from build123d import *

# Parameters (mm, degrees)
BOSS_EXTRU_1_DEPTH                                 = 14
BOSS_EXTRU_1_DEPTH_BACK                            = 7
ESQUISSE1_R                                        = 115
ESQUISSE1_R_2                                      = 10
ESQUISSE1_R_3                                      = 15.264337522
CHAMBRAGE_POUR_VIS_T_TE_HEXAGONALE_M12_D           = 13.5
CHAMBRAGE_POUR_VIS_T_TE_HEXAGONALE_M12_DEPTH       = 20
CHAMBRAGE_POUR_VIS_T_TE_HEXAGONALE_M12_CBORE_D     = 20
CHAMBRAGE_POUR_VIS_T_TE_HEXAGONALE_M12_CBORE_DEPTH = 12.6
CHAMBRAGE_POUR_VIS_T_TE_HEXAGONALE_M12_TIP         = 4.055809178
ECHELLE1_SCALE                                     = 0.25


with BuildPart() as part:
    # Esquisse1 → Boss.-Extru.1 (new, two sides: drawn at the far end of the back side and taken through both)
    with BuildSketch(Plane.XY.offset(-BOSS_EXTRU_1_DEPTH_BACK)):
        Circle(ESQUISSE1_R)
        with Locations((0, 72)):
            Circle(ESQUISSE1_R_2, mode=Mode.SUBTRACT)
        with Locations((-62.437871739, -35.854039838)):
            Circle(ESQUISSE1_R_2, mode=Mode.SUBTRACT)
        with Locations((62.269445197, -36.145763165)):
            Circle(ESQUISSE1_R_2, mode=Mode.SUBTRACT)
        Circle(ESQUISSE1_R_3, mode=Mode.SUBTRACT)
    extrude(amount=BOSS_EXTRU_1_DEPTH + BOSS_EXTRU_1_DEPTH_BACK)

    # Chambrage pour vis à tête hexagonale M121
    with Locations(Plane.XY.offset(14)):
        with Locations((0, -76.560659085), (65.614813045, 35.516704779), (-65.803859781, 40.113875083)):
            CounterBoreHole(CHAMBRAGE_POUR_VIS_T_TE_HEXAGONALE_M12_D / 2, CHAMBRAGE_POUR_VIS_T_TE_HEXAGONALE_M12_CBORE_D / 2, CHAMBRAGE_POUR_VIS_T_TE_HEXAGONALE_M12_CBORE_DEPTH, depth=CHAMBRAGE_POUR_VIS_T_TE_HEXAGONALE_M12_DEPTH)
            with Locations((0, 0, -(CHAMBRAGE_POUR_VIS_T_TE_HEXAGONALE_M12_DEPTH + CHAMBRAGE_POUR_VIS_T_TE_HEXAGONALE_M12_TIP / 2))):  # 118° drill point
                Cone(0, CHAMBRAGE_POUR_VIS_T_TE_HEXAGONALE_M12_D / 2, CHAMBRAGE_POUR_VIS_T_TE_HEXAGONALE_M12_TIP, mode=Mode.SUBTRACT)


with BuildPart() as part_1:
    # Echelle1: scaled about (0.002531385, 0.00580145, 3.465766244)
    add(part.part.scale(ECHELLE1_SCALE).moved(Location((0.001898539, 0.004351087, 2.599324683))))


solid = part_1.part
The model under review builds one solid part; all positions refer to its coordinate system, in mm. A direction names the side the tool comes from. Round coordinates to 2 decimals unless told otherwise and drop trailing zeros. Write each loop counter-clockwise with the first axis right and the second up, starting at its lowest first coordinate (ties: lowest second). Pieces come first, ordered by that corner, then holes. Notation, with made-up numbers: (-26.5, 12) - (2.5, 12) arc R25 cw to (2.5, 51) - close; hole circle Ø5 at (55, 83). An arc over 180 degrees is marked (long way). One line per item, written item: value. Start each with the question number.
1. Consider section C-C on x = 10. Write out the cut boundary in (y, z).
2. Consider section B-B on z = 2. State how many separate pieces and enclosed holes the cut face has, and give its area (3 significant figures).
3. The part is to be moulded in two halves that separate along X. For faces 1 (the face through (17, 7, 2.949)), 2 (the face through (6, 0, 6.099)), 3 (the face through (-3.74, 28.51, 3.44)), say which applies: released by +X, released by -X, zero draft, split by the parting line, or undercut.
4. To check wall thickness, follow L1, parallel to Y at x = -2, z = 2.9; L2, parallel to Y at x = 0.5, z = 4.4; L3, parallel to X at y = 20, z = 4.95. State the ranges of each line that lie inside material, in increasing order. Write a range as from..to.
5. Clearance check with flat-ended pins moving along their axes: P1, Ø1.5, axis at x = 16, z = 4.5, coming from the +Y side; P2, Ø2, axis at y = 9.5, z = 4, coming from the -X side; P3, Ø2.5, axis at x = -15.5, y = 10, coming from the +Z side. State where each tip first meets the part, or that it passes through.
6. Consider section D-D on y = -25. Write out the cut boundary in (x, z), and give its area (3 significant figures).
7. Machinability: for faces 4 (the face through (-18.06, 10.54, 2.01)), 5 (the face through (-0.83, -3.72, 3.44)), which of the approach directions +Z, -Z, +X, -X, +Y, -Y give a long, thin tool a straight path to every point of the face, cutting with its end or side? Answer none if there is none.
8. Consider section A-A on y = -2.5. Write out the cut boundary in (x, z).
Checks:
1. outline: (-26.95, 0.85) - (26.96, 0.85) - (26.96, 6.1) - (-26.95, 6.1) - close
2. separate pieces: 1
2. enclosed holes: 7
2. area: 2,470 mm^2
3. face 1: undercut
3. face 2: zero draft
3. face 3: split by the parting line
4. L1: y = -28.68..-3.24, 3.25..16.51, 19.5..28.68
4. L2: y = -28.74..-21.59, -16.69..-3.78, 3.79..15.55, 20.45..28.75
4. L3: x = -20.66..-1.5, 1.51..20.66
5. P1: stops at y = 24.38
5. P2: stops at x = -27.46
5. P3: stops at z = 2.95
6. outline: (-14.19, 0.85) - (14.19, 0.85) - (14.19, 6.1) - (-14.19, 6.1) - close
6. area: 149 mm^2
7. face 4: +Z
7. face 5: +Z, -Z
8. outline: (-28.64, 0.85) - (-2.88, 0.85) - (-2.88, 6.1) - (-28.64, 6.1) - close; (2.88, 0.85) - (28.64, 0.85) - (28.64, 6.1) - (2.88, 6.1) - close
